Part model, mm, in its own coordinate system. A direction names the side the tool comes from. Give positions to 0.01 mm unless a question says otherwise; leave off trailing zeros. Loops run counter-clockwise (first coordinate to the right, second up) from the corner with the lowest first, then second, coordinate; pieces in that order, holes last. Notation, with made-up numbers: (42.25, 14) -> (56.25, 14) arc R16 ccw to (56.25, 42) -> close; hole circle Ø10 at (14, 44). An arc over 180 degrees is marked (long way). One line per question, with ' | ' between items.
```python
from build123d import *

# Parameters (mm, degrees)
SKETCH2_W          = 10.8
SKETCH2_H          = 3
CUT_EXTRUDE1_START = -1.5
SKETCH3_R          = 1.7
CUT_EXTRUDE1_DEPTH = 1.5
SKETCH3_3_R        = 1.7
CUT_EXTRUDE2_DEPTH = 62.692059893


with BuildPart() as part:
    # Sketch2 → Revolve1 (revolve)
    with BuildSketch(Plane.XY, mode=Mode.PRIVATE) as revolve1_sk:
        Polygon((-24.056390036, 17.628606655), (-25.076178005, 17.628606655), (-27.076178005, 27.628606655), (-27.076178005, 30.628606655), (-26.656390036, 30.628606655), align=None)
        with Locations((-32.476178005, 29.128606655)):
            Rectangle(SKETCH2_W, SKETCH2_H)
    revolve(revolve1_sk.sketch.rotate(Axis((3.423821995, 17.628606655, 0), (0, 1, 0)), 270), axis=Axis((3.423821995, 17.628606655, 0), (0, 1, 0)))

    # Sketch3 → Cut-Extrude1 (cut)
    # profile 1 of 4: a face of its own
    with BuildSketch(Plane.XZ.offset(-27.628606655).offset(CUT_EXTRUDE1_START)):
        with BuildLine():
            Line((6.623821995, 35.5), (6.623821995, 41.175842432))
            ThreePointArc((6.623821995, 41.175842432), (3.423821995, 41.3), (0.223821995, 41.175842432))
            Line((0.223821995, 41.175842432), (0.223821995, 35.5))
            ThreePointArc((0.223821995, 35.5), (3.423821995, 32.3), (6.623821995, 35.5))
        make_face()
        with Locations(Location((3.423821995, 35.5, 0), (0, 0, 270))):
            Circle(SKETCH3_R, mode=Mode.SUBTRACT)
    # profile 2 of 4: a face of its own
    with BuildSketch(Plane.XZ.offset(-27.628606655).offset(CUT_EXTRUDE1_START)):
        with BuildLine():
            Line((38.923821995, -3.2), (44.599664427, -3.2))
            ThreePointArc((44.599664427, -3.2), (44.69277093, -1.601203852), (44.723821995, 0))
            ThreePointArc((44.723821995, 0), (44.69277093, 1.601203852), (44.599664427, 3.2))
            Line((44.599664427, 3.2), (38.923821995, 3.2))
            ThreePointArc((38.923821995, 3.2), (35.723821995, 0), (38.923821995, -3.2))
        make_face()
        with Locations(Location((38.923821995, 0, 0), (0, 0, 270))):
            Circle(SKETCH3_R, mode=Mode.SUBTRACT)
    # profile 3 of 4: a face of its own
    with BuildSketch(Plane.XZ.offset(-27.628606655).offset(CUT_EXTRUDE1_START)):
        with BuildLine():
            ThreePointArc((-37.752020437, 3.2), (-37.876178005, 0), (-37.752020437, -3.2))
            Line((-37.752020437, -3.2), (-32.076178005, -3.2))
            ThreePointArc((-32.076178005, -3.2), (-28.876178005, 0), (-32.076178005, 3.2))
            Line((-32.076178005, 3.2), (-37.752020437, 3.2))
        make_face()
        with Locations(Location((-32.076178005, 0, 0), (0, 0, 270))):
            Circle(SKETCH3_R, mode=Mode.SUBTRACT)
    # profile 4 of 4: a face of its own
    with BuildSketch(Plane.XZ.offset(-27.628606655).offset(CUT_EXTRUDE1_START)):
        with BuildLine():
            ThreePointArc((0.223821995, -41.175842432), (3.423821995, -41.3), (6.623821995, -41.175842432))
            Line((6.623821995, -41.175842432), (6.623821995, -35.5))
            ThreePointArc((6.623821995, -35.5), (3.423821995, -32.3), (0.223821995, -35.5))
            Line((0.223821995, -35.5), (0.223821995, -41.175842432))
        make_face()
        with Locations(Location((3.423821995, -35.5, 0), (0, 0, 270))):
            Circle(SKETCH3_R, mode=Mode.SUBTRACT)
    extrude(amount=CUT_EXTRUDE1_DEPTH, mode=Mode.SUBTRACT)

    # Sketch3_3 → Cut-Extrude2 (cut, through all)
    with BuildSketch(Plane.XZ.offset(-27.628606655)):
        with Locations(Location((3.423821995, 35.5, 0), (0, 0, 270))):
            Circle(SKETCH3_3_R)
        with Locations(Location((3.423821995, -35.5, 0), (0, 0, 270))):
            Circle(SKETCH3_3_R)
        with Locations(Location((-32.076178005, 0, 0), (0, 0, 270))):
            Circle(SKETCH3_3_R)
        with Locations(Location((38.923821995, 0, 0), (0, 0, 270))):
            Circle(SKETCH3_3_R)
    extrude(amount=-CUT_EXTRUDE2_DEPTH, mode=Mode.SUBTRACT)


solid = part.part
```
1) Drill centre lines: line 1 (X direction, y = 30.25, z = 0); line 2 (Y direction, x = 40, z = 3.5); line 3 (X direction, y = 29, z = 22). Where is each one in solid material? Low to high.
Found:
line 1: -37.88 to -33.78, -30.38 to -26.58, 33.43 to 37.22, 40.62 to 44.72 | line 2: 27.63 to 30.63 | line 3: -31.53 to -16.61, 23.46 to 38.38
2) Pull direction Z, two halves, no side cores. Call faces 1 (the cylindrical face through (-28.877, 28.389, -0.07)), 2 (the flat face through (-20, 17.629, -15)), 3 (the flat face through (41, 29.129, 0)), 4 (the cylindrical face through (3.4, 28.4, 32.3)): pulls with the +Z half, pulls with the -Z half, needs draft (parallel to the pull), parting line crosses it, or undercut.
Found:
face 1: undercut | face 2: needs draft | face 3: undercut | face 4: pulls with the +Z half
3) Pin check, flat tips, straight feed: P1, Ø0.8, axis at x = -34.5, y = 28.5, coming from the -Z side; P2, Ø0.8, axis at y = 28.5, z = -38.5, coming from the +X side; P3, Ø1.2, axis at x = 42, y = 28.5, coming from the +Z side. Stop position of each tip, or through.
Found:
P1: z = -17.25 | P2: x = 19.36 | P3: z = 16.23
4) Tool access for faces 5 (the cylindrical face through (3.5, 28.4, -32.3)), 6 (the flat face through (-21.2, 27.629, 18.5)), 7 (the flat face through (-34, 29.129, 0)): list every direction of +Z, -Z, +X, -X, +Y, -Y with a clear straight run to the whole face (end or side of a thin tool).
Found:
face 5: -Z, -Y | face 6: -Y | face 7: -X, -Y
5) Saw through at A-A (z = 0). Give the cut face in (x, y), and give its area (3 significant figures).
Found:
outline: (-37.88, 29.13) -> (-33.78, 29.13) -> (-33.78, 30.63) -> (-37.88, 30.63) -> close; (-30.38, 29.13) -> (-28.88, 29.13) -> (-28.88, 27.63) -> (-27.08, 27.63) -> (-25.08, 17.63) -> (-24.06, 17.63) -> (-26.66, 30.63) -> (-30.38, 30.63) -> close; (30.9, 17.63) -> (31.92, 17.63) -> (33.92, 27.63) -> (35.72, 27.63) -> (35.72, 29.13) -> (37.22, 29.13) -> (37.22, 30.63) -> (33.5, 30.63) -> close; (40.62, 29.13) -> (44.72, 29.13) -> (44.72, 30.63) -> (40.62, 30.63) -> close | area: 52.3 mm2
6) Saw through at C-C (y = 19). Give the cut face in (x, z), and give its area (3 significant figures).
Found:
outline: circle Ø57.55 at (3.42, 0); hole circle Ø55.51 at (3.42, 0) | area: 181 mm2
7) Saw through at B-B (y = 24). Give the cut face in (x, z).
Found:
outline: circle Ø59.55 at (3.42, 0); hole circle Ø57.51 at (3.42, 0)
